For this review, take the finished solid that the model builds, in its own axes (mm). A direction names the side the tool comes from. Coordinates: 2 decimals unless noted, no trailing zeros. Loops run counter-clockwise (first coordinate to the right, second up) from the corner with the lowest first, then second, coordinate; pieces in that order, holes last. Notation, with made-up numbers: M 43.25,35 L 100.25,35 A11 cw 100.25,49 Z; hole C -9.5,28.5 d8. An arc over 180 degrees is marked long. Answer as a JSON object with one key per item and string values. Group by question number.
Item 1: Mouldability with a two-part tool opening along Z and no side actions: class faces 6 (the face through (109, 91, 164)), 7 (the face through (525.1, 15.915, 178.62)), 8 (the face through (180, 91, -15)), 9 (the face through (180, 92, 83)) as +Z half, -Z half, draft (parallel to the pull), parting line (faces both ways), or undercut.
Item 2: Tool access review of faces 1 (the face through (180, 91, 180)), 2 (the face through (109, 91, 6)), 3 (the face through (109, 91, 0)), 4 (the face through (537.858, 168.232, 167.315)), 5 (the face through (880, 45, -26)): name each direction out of +Z, -Z, +X, -X, +Y, -Y from which nothing blocks a thin tool from reaching the whole face with its end or side.
Item 3: Wall thickness on L1, parallel to Y at x = 668.5, z = 82; L2, parallel to Y at x = 90, z = 160.9; L3, parallel to Z at x = 201, y = 94.5: over which ranges is each line inside the solid? List them lowest first. Write a range as from..to.
Item 4: Insertion check: pin 1 (2 mm diameter, centred on x = 599, z = 103, fed in from -Y); pin 2 (8 mm diameter, centred on x = 354.5, y = 166, fed in from -Z); pin 3 (3 mm diameter, centred on x = 140, z = 159.5, fed in from +Y). Each pin has a flat end and moves straight along its axis. Give the tip position at first contact, or say it passes through.
Item 5: Add section A-A (z = 82). State the section outline as (x, y) points, then the cut area to 3 significant figures.
Item 6: Add section C-C (y = 135.5). State the section outline as (x, z) points, then the cut area to 3 significant figures.
Item 7: Add section B-B (x = 272). State the section outline as (y, z) points.
Item 8: Add section D-D (z = -21.5). State the section outline as (x, y) points.
from build123d import *

# Parameters (mm, degrees)
IZIM1_W                     = 180
IZIM1_H                     = 180
Y_KSEKLIK_EKSTR_ZYON1_DEPTH = 164
IZIM3_R                     = 121.753850042
Y_KSEKLIK_EKSTR_ZYON2_DEPTH = 700
KES_EKSTR_ZYON1_DEPTH       = 700
IZIM5_W                     = 180
IZIM5_H                     = 152
KES_EKSTR_ZYON2_DEPTH       = 700
IZIM6_R                     = 5
KES_EKSTR_ZYON3_DEPTH       = 700
IZIM7_R                     = 115.753850042
KES_EKSTR_ZYON4_DEPTH       = 694


with BuildPart() as part:
    # Çizim1 → Yükseklik-Ekstrüzyon1 (new body)
    with BuildSketch(Plane.XY):
        with Locations((90, 90)):
            Rectangle(IZIM1_W, IZIM1_H)
    extrude(amount=Y_KSEKLIK_EKSTR_ZYON1_DEPTH)

    # Çizim3 → Yükseklik-Ekstrüzyon2 (add)
    with BuildSketch(Plane(origin=(180, 0, 0), x_dir=(0, 0, -1), z_dir=(1, 0, 0))):
        with Locations((-82, 90)):
            Circle(IZIM3_R)
    extrude(amount=Y_KSEKLIK_EKSTR_ZYON2_DEPTH)

    # Çizim4 → Kes-Ekstrüzyon1 (cut)
    with BuildSketch(Plane.XY.offset(164)):
        with BuildLine():
            ThreePointArc((0, 90), (26.360389693, 153.639610307), (90, 180))
            Line((90, 180), (0, 180))
            Line((0, 180), (0, 90))
        make_face()
        with BuildLine():
            ThreePointArc((90, 0), (26.360389693, 26.360389693), (0, 90))
            Line((0, 90), (0, 0))
            Line((0, 0), (90, 0))
        make_face()
    extrude(amount=-KES_EKSTR_ZYON1_DEPTH, mode=Mode.SUBTRACT)

    # Çizim5 → Kes-Ekstrüzyon2 (cut)
    with BuildSketch(Plane(origin=(0, 180, 0), x_dir=(1, 0, 0), z_dir=(0, 1, 0))):
        with Locations((90, -82)):
            Rectangle(IZIM5_W, IZIM5_H)
    extrude(amount=-KES_EKSTR_ZYON2_DEPTH, mode=Mode.SUBTRACT)

    # Çizim6 → Kes-Ekstrüzyon3 (cut)
    with BuildSketch(Plane.XY.offset(164)):
        with Locations((90, 90)):
            Circle(IZIM6_R)
    extrude(amount=-KES_EKSTR_ZYON3_DEPTH, mode=Mode.SUBTRACT)

    # Çizim7 → Kes-Ekstrüzyon4 (cut)
    with BuildSketch(Plane(origin=(880, 0, 0), x_dir=(0, 0, -1), z_dir=(1, 0, 0))):
        with Locations((-82, 90)):
            Circle(IZIM7_R)
    extrude(amount=-KES_EKSTR_ZYON4_DEPTH, mode=Mode.SUBTRACT)


solid = part.part
From the geometry:
{
 "1": {"face 6": "+Z half", "face 7": "parting line", "face 8": "draft", "face 9": "undercut"},
 "2": {"face 1": "+Z, -X, +Y, -Y", "face 2": "-X, +Y, -Y", "face 3": "-Z, -X, +Y, -Y", "face 4": "+X", "face 5": "+Z, -Z, +X, +Y, -Y"},
 "3": {"L1": "y = -31.75..-25.75, 205.75..211.75", "L2": "y = 0..85, 95..180", "L3": "z = -39.67..-33.67, 197.67..203.67"},
 "4": {"pin 1": "stops at y = -30.1", "pin 2": "stops at z = -16.18", "pin 3": "stops at y = 180"},
 "5": {"outline": "M 180,-31.75 L 880,-31.75 L 880,-25.75 L 186,-25.75 L 186,205.75 L 880,205.75 L 880,211.75 L 180,211.75 Z", "area": "9,790 mm²"},
 "6": {"outline": "M 12.35,0 L 180,0 L 180,-30.93 L 880,-30.93 L 880,-24.44 L 186,-24.44 L 186,188.44 L 880,188.44 L 880,194.93 L 180,194.93 L 180,164 L 12.35,164 L 12.35,158 L 180,158 L 180,6 L 12.35,6 Z", "area": "12,400 mm²"},
 "7": {"outline": "C 90,82 d243.51; hole C 90,82 d231.51"},
 "8": {"outline": "M 180,25.88 L 880,25.88 L 880,38.17 L 186,38.17 L 186,141.83 L 880,141.83 L 880,154.12 L 180,154.12 Z"}
}
